The listing builds one solid part. Answer for the finished solid, in the listing's coordinates (mm). Face numbers are marked on the shaded views. A direction names the side the tool comes from. Coordinates: 2 decimals unless noted, no trailing zeros. Write each loop counter-clockwise with the first axis right and the second up, starting at its lowest first coordinate (ties: lowest second). Pieces come first, ordered by that corner, then holes.
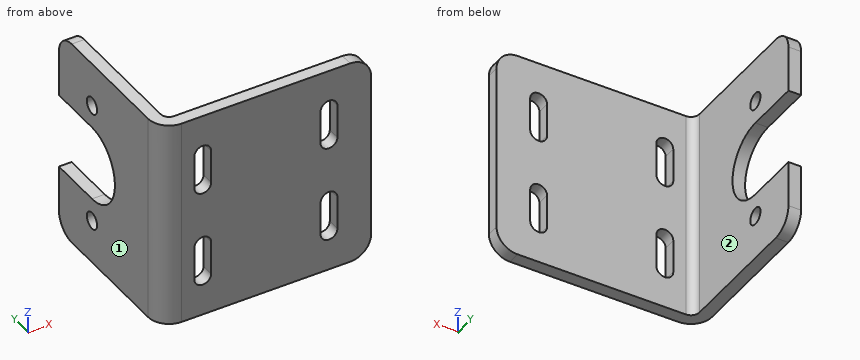
```python
from build123d import *

# Parameters (mm, degrees)
EXTRUDE_1_DEPTH     = 50
SKETCH_2_R          = 2
CUT_EXTRUDE_1_DEPTH = 3
CUT_EXTRUDE_2_DEPTH = 3
FILLET_1_R          = 5
FILLET_2_R          = 5


with BuildPart() as part:
    # 草图1 → 凸台-拉伸1 (new body)
    with BuildSketch(Plane.XY):
        with BuildLine():
            Line((0, 19.792207792), (0, -15.207792208))
            ThreePointArc((0, -15.207792208), (0.585786438, -16.62200577), (2, -17.207792208))
            Line((2, -17.207792208), (47, -17.207792208))
            Line((47, -17.207792208), (47, -20.207792208))
            Line((47, -20.207792208), (-3, -20.207792208))
            Line((-3, -20.207792208), (-3, 19.792207792))
            Line((-3, 19.792207792), (0, 19.792207792))
        make_face()
    extrude(amount=EXTRUDE_1_DEPTH)

    # 草图2 → 切除-拉伸1 (cut)
    with BuildSketch(Plane.ZY.offset(3)):
        with Locations((10.5, 6.792207792)):
            Circle(SKETCH_2_R)
        with BuildLine():
            Line((34, 19.792207792), (16, 19.792207792))
            Line((16, 19.792207792), (16, 6.792207792))
            ThreePointArc((16, 6.792207792), (25, -2.207792208), (34, 6.792207792))
            Line((34, 6.792207792), (34, 19.792207792))
        make_face()
        with Locations((39.5, 6.792207792)):
            Circle(SKETCH_2_R)
    extrude(amount=-CUT_EXTRUDE_1_DEPTH, mode=Mode.SUBTRACT)

    # 草图3 → 切除-拉伸2 (cut)
    with BuildSketch(Plane.XZ.offset(20.207792208)):
        with BuildLine():
            Line((39, 32.5), (39, 40.5))
            ThreePointArc((39, 40.5), (37, 42.5), (35, 40.5))
            Line((35, 40.5), (35, 32.5))
            ThreePointArc((35, 32.5), (37, 30.5), (39, 32.5))
        make_face()
        with BuildLine():
            Line((35, 17.5), (35, 9.5))
            ThreePointArc((35, 9.5), (37, 7.5), (39, 9.5))
            Line((39, 9.5), (39, 17.5))
            ThreePointArc((39, 17.5), (37, 19.5), (35, 17.5))
        make_face()
        with BuildLine():
            Line((5, 17.5), (5, 9.5))
            ThreePointArc((5, 9.5), (7, 7.5), (9, 9.5))
            Line((9, 9.5), (9, 17.5))
            ThreePointArc((9, 17.5), (7, 19.5), (5, 17.5))
        make_face()
        with BuildLine():
            Line((9, 32.5), (9, 40.5))
            ThreePointArc((9, 40.5), (7, 42.5), (5, 40.5))
            Line((5, 40.5), (5, 32.5))
            ThreePointArc((5, 32.5), (7, 30.5), (9, 32.5))
        make_face()
    extrude(amount=-CUT_EXTRUDE_2_DEPTH, mode=Mode.SUBTRACT)

    # 圆角1
    fillet_1_edges = [part.edges().sort_by_distance(p)[0] for p in [
        (-3, -20.207792208, 25),
    ]]
    fillet(fillet_1_edges, radius=FILLET_1_R)

    # 圆角2
    fillet_2_edges = [part.edges().sort_by_distance(p)[0] for p in [
        (47, -18.707792208, 50),
        (-1.5, 19.792207792, 50),
        (47, -18.707792208, 0),
        (-1.5, 19.792207792, 0),
    ]]
    fillet(fillet_2_edges, radius=FILLET_2_R)


solid = part.part
```
(1) Each of these flat-tipped pins is pushed along its axis until it touches: pin 1 (22.5 mm diameter, centred on x = 32, z = 20, fed in from +Y); pin 2 (1.5 mm diameter, centred on y = -18.5, z = 13, fed in from -X); pin 3 (0.9 mm diameter, centred on y = -19, z = 15.5, fed in from -X). Where does it stop, or does it pass through?
(2) Section A-A, the plane y = 12 is taken. Write down the section's boundary in (x, z).
(3) Find the intervals of material crossed by probe 1 along Y at (x, z) = (42.5, 18); probe 2 along X at (y, z) = (-5.5, 37.5); probe 3 along Y at (x, z) = (-1, 10), in increasing order.
(4) Which of the six approach directions +Z, -Z, +X, -X, +Y, -Y give full straight-line access (tool end or side, diameter ignored) to the marked faces 1 and 2?
(5) Section D-D, the plane z = 25 is taken. Write down the section's boundary in (x, y).
(6) Section B-B, the plane z = 10.5 is taken. Write down the section's boundary in (x, y).
(7) Section C-C, the plane x = 7 is taken. Write down the section's boundary in (y, z).
Solution:
1. pin 1: stops at y = -17.21
1. pin 2: stops at x = -2.31
1. pin 3: stops at x = -1.72
2. outline: (-3, 0) - (0, 0) - (0, 16) - (-3, 16) - close; (-3, 34) - (0, 34) - (0, 50) - (-3, 50) - close
3. probe 1: y = -20.21 to -17.21
3. probe 2: x = -3 to 0
3. probe 3: y = -19.21 to 4.86, 8.73 to 19.79
4. face 1: +Z, -Z, -X, +Y, -Y
4. face 2: +Z, -Z, +X, +Y
5. outline: (-3, -15.21) arc R5 ccw to (2, -20.21) - (47, -20.21) - (47, -17.21) - (2, -17.21) arc R2 cw to (0, -15.21) - (0, -2.21) - (-3, -2.21) - close
6. outline: (-3, -15.21) arc R5 ccw to (2, -20.21) - (5, -20.21) - (5, -17.21) - (2, -17.21) arc R2 cw to (0, -15.21) - (0, 4.79) - (-3, 4.79) - close; (-3, 8.79) - (0, 8.79) - (0, 19.79) - (-3, 19.79) - close; (9, -20.21) - (35, -20.21) - (35, -17.21) - (9, -17.21) - close; (39, -20.21) - (47, -20.21) - (47, -17.21) - (39, -17.21) - close
7. outline: (-20.21, 0) - (-17.21, 0) - (-17.21, 7.5) - (-20.21, 7.5) - close; (-20.21, 19.5) - (-17.21, 19.5) - (-17.21, 30.5) - (-20.21, 30.5) - close; (-20.21, 42.5) - (-17.21, 42.5) - (-17.21, 50) - (-20.21, 50) - close
